from build123d import *

# Parameters (mm, degrees)
F0_R     = 50
F1_DEPTH = 650
F2_R     = 46
F3_DEPTH = 26


with BuildPart() as f1:
    # F0 (on Right) → F1 (new body)
    with BuildSketch(Plane.YZ):
        Circle(F0_R)
        with BuildLine():
            ThreePointArc((26.59066, -35.056195), (16.838071, -40.650699), (5.986037, -43.590909))
            ThreePointArc((5.986037, -43.590909), (0, -38), (-5.986037, -43.590909))
            ThreePointArc((-5.986037, -43.590909), (-16.838071, -40.650699), (-26.59066, -35.056195))
            ThreePointArc((-26.59066, -35.056195), (-26.870058, -26.870058), (-35.056195, -26.59066))
            ThreePointArc((-35.056195, -26.59066), (-40.650699, -16.838071), (-43.590909, -5.986037))
            ThreePointArc((-43.590909, -5.986037), (-38, 0), (-43.590909, 5.986037))
            ThreePointArc((-43.590909, 5.986037), (-40.650699, 16.838071), (-35.056195, 26.59066))
            ThreePointArc((-35.056195, 26.59066), (-26.870058, 26.870058), (-26.59066, 35.056195))
            ThreePointArc((-26.59066, 35.056195), (-16.838071, 40.650699), (-5.986037, 43.590909))
            ThreePointArc((-5.986037, 43.590909), (0, 38), (5.986037, 43.590909))
            ThreePointArc((5.986037, 43.590909), (16.838071, 40.650699), (26.59066, 35.056195))
            ThreePointArc((26.59066, 35.056195), (26.870058, 26.870058), (35.056195, 26.59066))
            ThreePointArc((35.056195, 26.59066), (40.650699, 16.838071), (43.590909, 5.986037))
            ThreePointArc((43.590909, 5.986037), (38, 0), (43.590909, -5.986037))
            ThreePointArc((43.590909, -5.986037), (40.650699, -16.838071), (35.056195, -26.59066))
            ThreePointArc((35.056195, -26.59066), (26.870058, -26.870058), (26.59066, -35.056195))
        make_face(mode=Mode.SUBTRACT)
    extrude(amount=-F1_DEPTH)

    # F2 (on Right) → F3 (cut)
    with BuildSketch(Plane.YZ):
        Circle(F2_R)
    extrude(amount=-F3_DEPTH, mode=Mode.SUBTRACT)

    # F4: F1 across face


with BuildPart() as f1_1:
    add(f1.part)
    add(f1.part.mirror(Plane(origin=(-650, 0, 0), x_dir=(0, 1, 0), z_dir=(-1, 0, 0))))


solid = f1_1.part
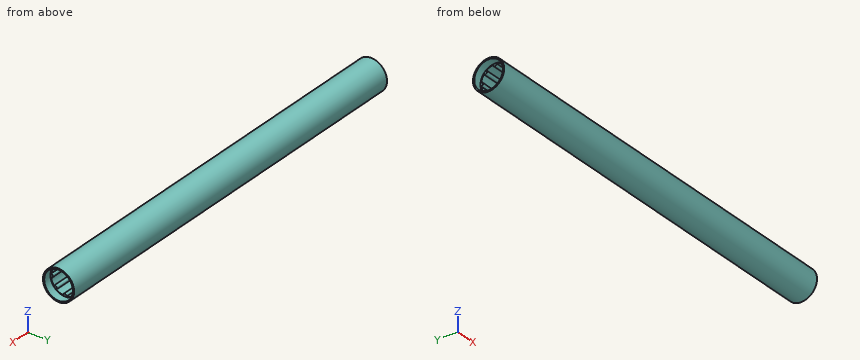
Input: part model. Units: mm. Frame: model coordinates. Give positions to 0.01 mm unless a question says otherwise; leave off trailing zeros. Write each loop counter-clockwise with the first axis right and the second up, starting at its lowest first coordinate (ties: lowest second). Pieces come first, ordered by that corner, then holes.
Q1. Section A-A, the plane x = -619. Output: boundary loops of the cut face in (y, z), plus the area to 3 significant figures.
Q2. First-contact query: P1, Ø5, axis at x = -1143.5, y = 22.5, coming from the -Z side; P2, Ø5, axis at x = -144, z = -33, coming from the +Y side; P3, Ø12, axis at x = -171.5, z = -33.5, coming from the +Y side. Flat tips, straight axial feed; report the tip coordinate or a pass-through.
Q3. Material intervals for probe 1 along Z at (x, y) = (-606, -1.5); probe 2 along Z at (x, y) = (-379.5, 37.5); probe 3 along Z at (x, y) = (-83, 26), sorted ascending.
Filled in:
1. outline: circle Ø100 at (0, 0); hole (-43.59, -5.99) arc R44 ccw to (-35.06, -26.59) arc R6 cw to (-26.59, -35.06) arc R44 ccw to (-5.99, -43.59) arc R6 cw to (5.99, -43.59) arc R44 ccw to (26.59, -35.06) arc R6 cw to (35.06, -26.59) arc R44 ccw to (43.59, -5.99) arc R6 cw to (43.59, 5.99) arc R44 ccw to (35.06, 26.59) arc R6 cw to (26.59, 35.06) arc R44 ccw to (5.99, 43.59) arc R6 cw to (-5.99, 43.59) arc R44 ccw to (-26.59, 35.06) arc R6 cw to (-35.06, 26.59) arc R44 ccw to (-43.59, 5.99) arc R6 cw to start
1. area: 2,210 mm2
2. P1: stops at z = -45.83
2. P2: stops at y = 39.62
2. P3: stops at y = 41.76
3. probe 1: z = -49.98 to -38.19, 38.19 to 49.98
3. probe 2: z = -33.07 to -23.02, 23.02 to 33.07
3. probe 3: z = -42.71 to -35.5, -34.25 to -27.97, 27.97 to 34.25, 35.5 to 42.71
